Read the model definition and answer for the solid it produces. Units are mm, in the model's axes. Coordinates: 2 decimals unless noted, no trailing zeros. Write each loop counter-clockwise with the first axis right and the second up, starting at its lowest first coordinate (ties: lowest second). Pieces come first, ordered by that corner, then holes.
Item 1: Section A-A (x = -31) is taken. Give the vertices of the cut face in (y, z), then the cut area to 3 significant figures.
Item 2: Section B-B (y = 0) is taken. Give the vertices of the cut face in (x, z).
Item 3: This flat-tipped pin is pushed along its axis until it touches: P1, Ø2, axis at x = -32.5, y = 1, coming from the +Z side. Where does it stop, or does it pass through?
Item 4: Straight lines are drawn through the part: probe 1 along X at (y, z) = (0.15, 1.95); probe 2 along Y at (x, z) = (-50, 1.6); probe 3 along X at (y, z) = (0.7, 1.35). For each, find the intervals that lie inside material, in ascending order.
Item 5: Section C-C (z = 1.3) is taken. Give the vertices of the cut face in (x, y).
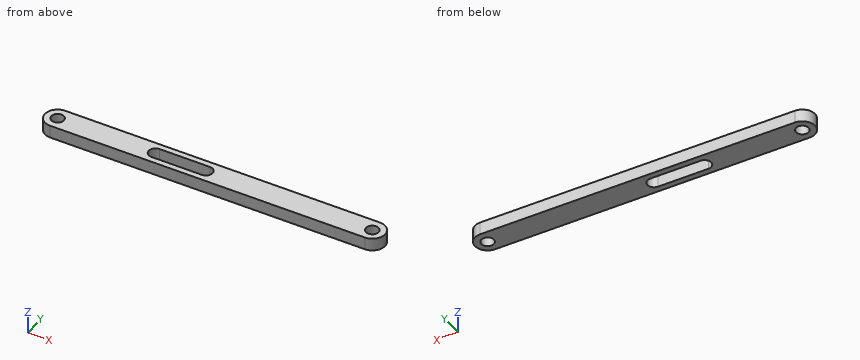
from build123d import *

# Parameters (mm, degrees)
SKETCH_R  = 1
PAD_DEPTH = 2


with BuildPart() as part:
    # Sketch → Pad (new body)
    with BuildSketch(Plane.XY):
        with BuildLine():
            ThreePointArc((-50, 2), (-52, 0), (-50, -2))
            Line((-50, -2), (0, -2))
            ThreePointArc((0, -2), (2, 0), (0, 2))
            Line((-50, 2), (0, 2))
        make_face()
        Circle(SKETCH_R, mode=Mode.SUBTRACT)
        with Locations((-50, 0)):
            Circle(SKETCH_R, mode=Mode.SUBTRACT)
        with BuildLine():
            ThreePointArc((-34.455448, 1.061365), (-35.516813, 0), (-34.455448, -1.061365))
            Line((-34.455448, -1.061365), (-26.442669, -1.061365))
            ThreePointArc((-26.442669, -1.061365), (-25.381304, 0), (-26.442669, 1.061365))
            Line((-34.455448, 1.061365), (-26.442669, 1.061365))
        make_face(mode=Mode.SUBTRACT)
    extrude(amount=PAD_DEPTH)


solid = part.part
Established:
1. outline: (-2, 0) - (-1.06, 0) - (-1.06, 2) - (-2, 2) - close; (1.06, 0) - (2, 0) - (2, 2) - (1.06, 2) - close
1. area: 3.75 mm2
2. outline: (-52, 0) - (-51, 0) - (-51, 2) - (-52, 2) - close; (-49, 0) - (-35.52, 0) - (-35.52, 2) - (-49, 2) - close; (-25.38, 0) - (-1, 0) - (-1, 2) - (-25.38, 2) - close; (1, 0) - (2, 0) - (2, 2) - (1, 2) - close
3. P1: stops at z = 2
4. probe 1: x = -51.99 to -50.99, -49.01 to -35.51, -25.39 to -0.99, 0.99 to 1.99
4. probe 2: y = -2 to -1, 1 to 2
4. probe 3: x = -51.87 to -50.71, -49.29 to -35.25, -25.64 to -0.71, 0.71 to 1.87
5. outline: (-50, -2) - (0, -2) arc R2 ccw to (0, 2) - (-50, 2) arc R2 ccw to start; hole circle Ø2 at (-50, 0); hole (-34.46, -1.06) - (-26.44, -1.06) arc R1.06 ccw to (-26.44, 1.06) - (-34.46, 1.06) arc R1.06 ccw to start; hole circle Ø2 at (0, 0)
